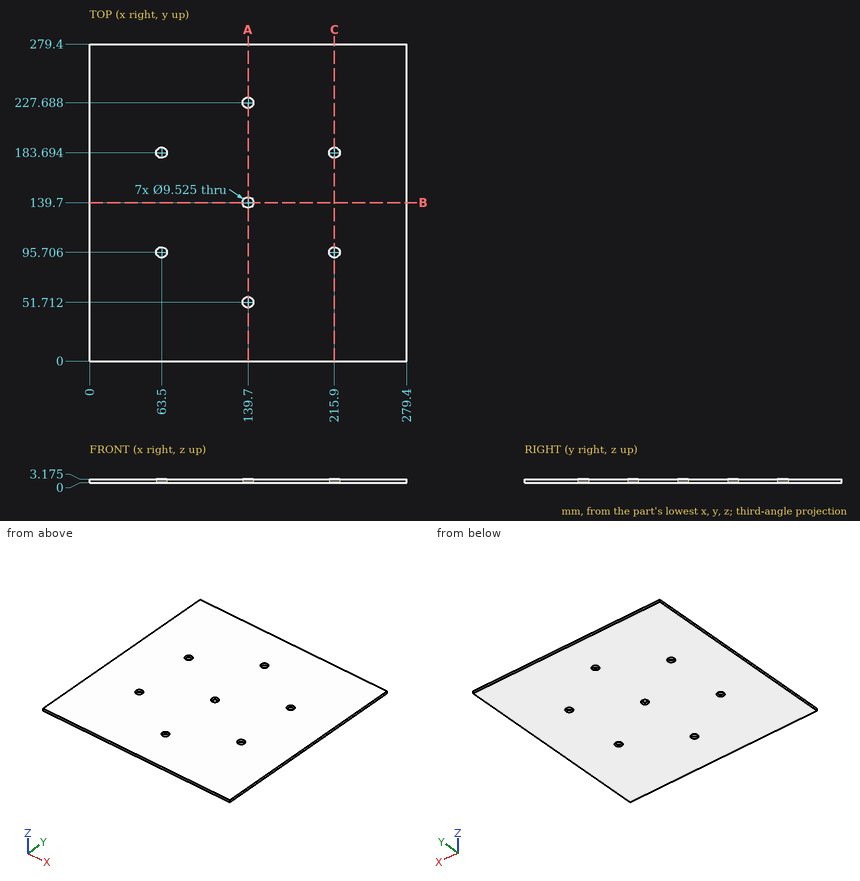
Answer from the drawing. Dimensions are ordinates in mm from the lowest x, y and z of the part. Coordinates: 2 decimals unless noted, no trailing zeros. Loops run counter-clockwise (first coordinate to the right, second up) from the corner with the lowest first, then second, coordinate; pieces in that order, holes last. Notation, with made-up numbers: (10, -39) -> (18, -39) arc R34 ccw to (18, -7) -> close; hole circle Ø4 at (83, 15.25). An arc over 180 degrees is marked (long way). Answer in a Markdown table with one row per item.
Item 1: A cutting plane is placed at C-C on x = 215.9. Determine the outline of the cut face in (y, z) (1 decimal).
Returned:
| item | result |
|---|---|
| outline | (0, 0) -> (90.9, 0) -> (90.9, 3.2) -> (0, 3.2) -> close; (100.5, 0) -> (178.9, 0) -> (178.9, 3.2) -> (100.5, 3.2) -> close; (188.5, 0) -> (279.4, 0) -> (279.4, 3.2) -> (188.5, 3.2) -> close |
Item 2: A cutting plane is placed at B-B on y = 139.7. Determine the outline of the cut face in (x, z) (1 decimal).
Returned:
| item | result |
|---|---|
| outline | (0, 0) -> (134.9, 0) -> (134.9, 3.2) -> (0, 3.2) -> close; (144.5, 0) -> (279.4, 0) -> (279.4, 3.2) -> (144.5, 3.2) -> close |
Item 3: A cutting plane is placed at A-A on x = 139.7. Determine the outline of the cut face in (y, z) (1 decimal).
Returned:
| item | result |
|---|---|
| outline | (0, 0) -> (46.9, 0) -> (46.9, 3.2) -> (0, 3.2) -> close; (56.5, 0) -> (134.9, 0) -> (134.9, 3.2) -> (56.5, 3.2) -> close; (144.5, 0) -> (222.9, 0) -> (222.9, 3.2) -> (144.5, 3.2) -> close; (232.5, 0) -> (279.4, 0) -> (279.4, 3.2) -> (232.5, 3.2) -> close |
Item 4: This flat-tipped pin is pushed along its axis until it touches: P1, Ø5.5, axis at x = 139.7, y = 51.71, coming from the +Z side. Where does it stop, or does it pass through?
Returned:
| item | result |
|---|---|
| P1 | passes through |
Item 5: Straight lines are drawn through the part: line 1 along Y through (x, z) = (215.9, 1.2); line 2 along Y through (x, z) = (139.7, 2.2); line 3 along Y through (x, z) = (215, 2.2). For each, find the intervals that lie inside material, in ascending order. Write a range as [from, to].
Returned:
| item | result |
|---|---|
| line 1 | y = [0, 90.94], [100.47, 178.93], [188.46, 279.4] |
| line 2 | y = [0, 46.95], [56.47, 134.94], [144.46, 222.93], [232.45, 279.4] |
| line 3 | y = [0, 91.03], [100.38, 179.02], [188.37, 279.4] |
